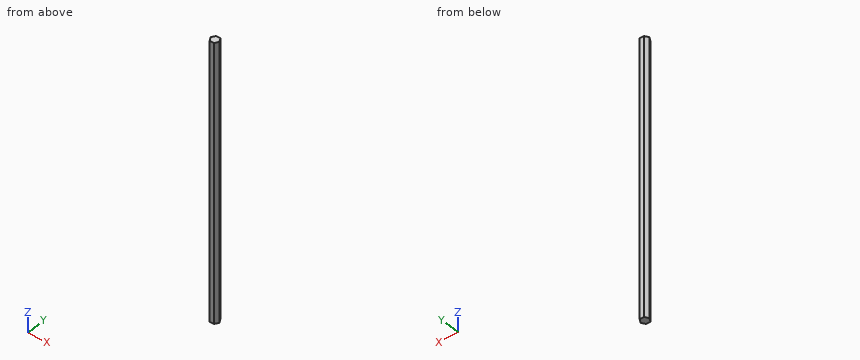
Autodesk Inventor part; units mm, degrees
ref_plane "YZ Plane" through (0, 0, 0) normal (1, 0, 0) x (0, 1, 0)
ref_plane "XZ Plane" through (0, 0, 0) normal (0, 1, 0) x (-1, 0, 0)
sketch "Sketch1" plane through (0, 0, 0) normal (0, 0, 1) x (1, 0, 0)
  line L0 (7.3323, 0) -> (3.6662, -6.35)
  line L1 (3.6662, -6.35) -> (-3.6662, -6.35)
  line L2 (-3.6662, -6.35) -> (-7.3323, 0)
  line L3 (-7.3323, 0) -> (-3.6662, 6.35)
  line L4 (-3.6662, 6.35) -> (3.6662, 6.35)
  line L5 (3.6662, 6.35) -> (7.3323, 0)
  point P0 (0, 0)
  point P1 (0, 0)
  dimension "d0" = 12.7
extrude "Extrusion1" add sketch "Sketch1" along normal mid plane 457.2
properties part number "hexExtrusion"
Geometry check sheet. Reference: the model listing, model coordinates, mm. Give positions to 0.01 mm unless a question says otherwise; leave off trailing zeros. Write each loop counter-clockwise with the first axis right and the second up, starting at its lowest first coordinate (ties: lowest second). Pieces come first, ordered by that corner, then holes. Notation, with made-up numbers: (-30, -13) -> (-15, -13) arc R18 ccw to (-15, -2) -> close; hole circle Ø9 at (71.25, 68.5). An arc over 180 degrees is marked (long way). Use one line per item in the form item = value.
Item 1: Sectioned sample at B-B on y = 3.25. Enter the section's corners in (x, z).
Results list:
outline = (-5.46, -228.6) -> (5.46, -228.6) -> (5.46, 228.6) -> (-5.46, 228.6) -> close
Item 2: Depth check by flat-ended pin: pin 1 Ø1 at (y, z) = (1, 42) entering from -X; pin 2 Ø2 at (x, z) = (-5, -11) entering from -Y; pin 3 Ø1.5 at (y, z) = (-3.5, -88) entering from -X. Enter the tip coordinate at first touch or a pass-through.
Results list:
pin_1 = -7.04
pin_2 = -5.77
pin_3 = -5.74
Item 3: Scan lines: line 1 (X direction, y = 1.75, z = -197.5); line 2 (X direction, y = -1.5, z = 40.5); line 3 (Y direction, x = -4.75, z = -64). Record each from-to range of solid material in increasing order.
Results list:
line_1 = -6.32 to 6.32
line_2 = -6.47 to 6.47
line_3 = -4.47 to 4.47
Item 4: Sectioned sample at A-A on z = 179.5. Enter the section's corners in (x, y), plus the area to 3 significant figures.
Results list:
outline = (-7.33, 0) -> (-3.67, -6.35) -> (3.67, -6.35) -> (7.33, 0) -> (3.67, 6.35) -> (-3.67, 6.35) -> close
area = 140 mm2
